from build123d import *

# Parameters (mm, degrees)
PAD007_DEPTH    = 14.7
PAD008_DEPTH    = 8.5
POCKET017_DEPTH = 7.22
SKETCH022_R     = 7.7
POCKET018_DEPTH = 26.5
SKETCH023_R     = 7.7
POCKET019_DEPTH = 26
SKETCH024_R     = 6
SKETCH024_R_2   = 5.5
POCKET020_DEPTH = 57.001
SKETCH025_R     = 7.7
POCKET021_DEPTH = 26
SKETCH020_W     = 25.7447
SKETCH020_H     = 35
POCKET022_DEPTH = 2.2
FILLET_R        = 1
FILLET001_R     = 1
FILLET002_R     = 2
SKETCH026_R     = 1.55
SKETCH026_R_2   = 1.6
POCKET023_DEPTH = 14.701
SKETCH027_R     = 1.55
POCKET024_DEPTH = 23.201
SKETCH028_R     = 1.55
POCKET025_DEPTH = 10
SKETCH029_W     = 10
SKETCH029_H     = 57
PAD009_DEPTH    = 9.5
POCKET026_DEPTH = 16.981
SKETCH031_W     = 10
SKETCH031_H     = 2.9
POCKET027_DEPTH = 1.5
POCKET028_DEPTH = 10
SKETCH033_R     = 1.7
POCKET029_DEPTH = 16
SKETCH_W        = 6
SKETCH_H        = 3
POCKET_DEPTH    = 23.201


with BuildPart() as part:
    # Sketch018 → Pad007 (new body)
    with BuildSketch(Plane.YZ):
        Polygon((0, 0), (0, 26), (-4.306836, 40.539634), (3.9, 57), (74.5, 57), (74.5, 0), align=None)
    extrude(amount=PAD007_DEPTH)

    # Sketch019 → Pad008 (new body)
    with BuildSketch(Plane.YZ.offset(14.7)):
        Polygon((19.7447, 57), (28.4947, 57), (28.4947, 12.3), (21.6234, 12.3), (21.6234, 26.5), (19.7447, 26.5), align=None)
    extrude(amount=PAD008_DEPTH)

    # Sketch021 → Pocket017 (cut)
    with BuildSketch(Plane.YZ.offset(14.7)):
        with BuildLine():
            ThreePointArc((44.6197, 57), (41.229345, 42.566333), (43.9947, 28))
            Line((43.9947, -6), (43.9947, 28))
            Line((43.9947, -6), (28.4947, -6))
            Line((28.4947, -6), (28.4947, 65))
            Line((28.4947, 65), (44.6197, 65))
            Line((44.6197, 65), (44.6197, 57))
        make_face()
    extrude(amount=-POCKET017_DEPTH, mode=Mode.SUBTRACT)

    # Sketch022 → Pocket018 (cut)
    with BuildSketch(Plane.YX):
        with Locations((14.25, 12.5)):
            Circle(SKETCH022_R)
    extrude(amount=-POCKET018_DEPTH, mode=Mode.SUBTRACT)

    # Sketch023 → Pocket019 (cut)
    with BuildSketch(Plane.YX):
        with Locations((59.25, 12.5)):
            Circle(SKETCH023_R)
    extrude(amount=-POCKET019_DEPTH, mode=Mode.SUBTRACT)

    # Sketch024 → Pocket020 (cut, through all)
    with BuildSketch(Plane(origin=(0, 0, 57), x_dir=(0, -1, 0), z_dir=(0, 0, 1))):
        with Locations((-59.25, 12.5)):
            Circle(SKETCH024_R)
        with Locations((-14.25, 12.5)):
            Circle(SKETCH024_R_2)
    extrude(amount=-POCKET020_DEPTH, mode=Mode.SUBTRACT)

    # Sketch025 → Pocket021 (cut)
    with BuildSketch(Plane(origin=(0, 0, 57), x_dir=(0, -1, 0), z_dir=(0, 0, 1))):
        with Locations((-59.25, 12.5)):
            Circle(SKETCH025_R)
    extrude(amount=-POCKET021_DEPTH, mode=Mode.SUBTRACT)

    # Sketch020 → Pocket022 (cut)
    with BuildSketch(Plane.YZ.offset(14.7)):
        with Locations((6.87235, 43.5)):
            Rectangle(SKETCH020_W, SKETCH020_H)
    extrude(amount=-POCKET022_DEPTH, mode=Mode.SUBTRACT)

    # Fillet
    fillet_edges = [part.edges().sort_by_distance(p)[0] for p in [
        (7.001325, 14.370727, 57),
        (7.001325, 14.370727, 26.5),
    ]]
    fillet(fillet_edges, radius=FILLET_R)

    # Fillet001
    fillet001_edges = [part.edges().sort_by_distance(p)[0] for p in [
        (6.25, 3.9, 57),
        (12.5, 5.825, 57),
        (12.5, -0.203418, 48.769817),
        (6.25, -4.306836, 40.539634),
        (12.5, -2.153418, 33.269817),
    ]]
    fillet(fillet001_edges, radius=FILLET001_R)

    # Fillet002
    fillet002_edges = [part.edges().sort_by_distance(p)[0] for p in [
        (7.35, 0, 0),
        (18.959389, 21.6234, 12.3),
        (11.09, 43.9947, 0),
        (11.09, 28.4947, 0),
        (7.35, 74.5, 0),
        (7.35, 74.5, 57),
        (11.09, 28.4947, 57),
        (18.95, 28.4947, 57),
    ]]
    fillet(fillet002_edges, radius=FILLET002_R)

    # Sketch026 → Pocket023 (cut, through all)
    with BuildSketch(Plane.YZ.offset(14.7)):
        with Locations((2, 40)):
            Circle(SKETCH026_R)
        with Locations((3.5, 19.8)):
            Circle(SKETCH026_R_2)
        with Locations((25, 6.2)):
            Circle(SKETCH026_R_2)
        with Locations((48.3, 44)):
            Circle(SKETCH026_R_2)
        with Locations((48.3, 13)):
            Circle(SKETCH026_R_2)
        with Locations((70.2, 44)):
            Circle(SKETCH026_R_2)
        with Locations((70.2, 13)):
            Circle(SKETCH026_R_2)
    extrude(amount=-POCKET023_DEPTH, mode=Mode.SUBTRACT)

    # Sketch027 → Pocket024 (cut, through all)
    with BuildSketch(Plane.YZ.offset(23.2)):
        with Locations((25, 40)):
            Circle(SKETCH027_R)
        with Locations((25, 17)):
            Circle(SKETCH027_R)
    extrude(amount=-POCKET024_DEPTH, mode=Mode.SUBTRACT)

    # Sketch028 → Pocket025 (cut)
    with BuildSketch(Plane(origin=(0, 19.7447, 0), x_dir=(0, 0, -1), z_dir=(0, -1, 0))):
        with Locations((-50.5, 19)):
            Circle(SKETCH028_R)
        with Locations((-31.5, 19)):
            Circle(SKETCH028_R)
    extrude(amount=-POCKET025_DEPTH, mode=Mode.SUBTRACT)

    # Sketch029 → Pad009 (new body)
    with BuildSketch(Plane.YZ.offset(7.48)):
        with Locations((35, 28.5)):
            Rectangle(SKETCH029_W, SKETCH029_H)
    extrude(amount=PAD009_DEPTH)

    # Sketch030 → Pocket026 (cut, through all)
    with BuildSketch(Plane.YZ.offset(16.98)):
        with BuildLine():
            Line((30, 49), (30, 57))
            Line((30, 57), (40, 57))
            Line((40, 57), (40, 49))
            Line((38.5, 49), (40, 49))
            ThreePointArc((35.5, 49), (37, 47.5), (38.5, 49))
            Line((34.5, 49), (35.5, 49))
            ThreePointArc((31.5, 49), (33, 47.5), (34.5, 49))
            Line((30, 49), (31.5, 49))
        make_face()
    extrude(amount=-POCKET026_DEPTH, mode=Mode.SUBTRACT)

    # Sketch031 → Pocket027 (cut)
    with BuildSketch(Plane(origin=(0, 0, 49), x_dir=(0, -1, 0), z_dir=(0, 0, 1))):
        with Locations((-35, 1.45)):
            Rectangle(SKETCH031_W, SKETCH031_H)
    extrude(amount=-POCKET027_DEPTH, mode=Mode.SUBTRACT)

    # Sketch032 → Pocket028 (cut)
    with BuildSketch(Plane.ZX.offset(40)):
        Polygon((0, 7.48), (0, 16.98), (47, 16.98), (35.678341, 7.48), align=None)
    extrude(amount=-POCKET028_DEPTH, mode=Mode.SUBTRACT)

    # Sketch033 → Pocket029 (cut)
    with BuildSketch(Plane(origin=(0, 0, 49), x_dir=(0, -1, 0), z_dir=(0, 0, 1))):
        with Locations((-35, 5.41526)):
            Circle(SKETCH033_R)
    extrude(amount=-POCKET029_DEPTH, mode=Mode.SUBTRACT)

    # Sketch → Pocket (cut, through all)
    with BuildSketch(Plane(origin=(0, 0, 0), x_dir=(0, 1, 0), z_dir=(-1, 0, 0))):
        with Locations((35, -40.5)):
            Rectangle(SKETCH_W, SKETCH_H)
    extrude(amount=-POCKET_DEPTH, mode=Mode.SUBTRACT)


solid = part.part
The listing builds one solid part. Answer for the finished solid, in the listing's coordinates (mm). A direction names the side the tool comes from. Round coordinates to 2 decimals unless told otherwise and drop trailing zeros. Loops run counter-clockwise (first coordinate to the right, second up) from the corner with the lowest first, then second, coordinate; pieces in that order, holes last. Notation, with made-up numbers: M 6,-16.75 L 56,-16.75 A23 cw 56,2.25 Z; hole C 79,64 d3. An arc over 180 degrees is marked long. Return JSON: item names as keys, results as strings.
Q1. The mould has two halves that part along Z. Classify faces 4 (the face through (10, 37, 47.5)), 5 (the face through (23.2, 24, 35)), 6 (the face through (7.45, 23.82, 7.28)): released by +Z, released by -Z, zero draft, split by the parting line, or undercut.
Results list:
{"face 4": "released by +Z", "face 5": "zero draft", "face 6": "undercut"}
Q2. Find the intervals of material crossed by line 1 along Z through (x, y) = (11.5, 70.2); line 2 along Z through (x, y) = (5.5, 33); line 3 along X through (y, z) = (3, 38.5), in increasing order. Write a range as from..to.
Results list:
{"line 1": "z = 0..11.4, 14.6..42.4, 45.6..57", "line 2": "z = 0..39, 42..47.5", "line 3": "x = 0..12.5"}
Q3. Each of these flat-tipped pins is pushed along its axis until it touches: pin 1 Ø3 at (x, z) = (20.5, 42) entering from +Y; pin 2 Ø3.5 at (y, z) = (3, 37.5) entering from +X; pin 3 Ø3 at (y, z) = (25, 6.2) entering from -X; pin 4 Ø4 at (y, z) = (29.5, 38) entering from +X. Where does it stop, or does it pass through?
Results list:
{"pin 1": "stops at y = 28.49", "pin 2": "stops at x = 12.5", "pin 3": "passes through", "pin 4": "stops at x = 23.2"}
Q4. Find section B-B, the plane y = 25. Determine the outline of the cut face in (x, z), plus the area to 3 significant figures.
Results list:
{"outline": "M 0,0 L 14.7,0 L 14.7,4.6 L 0,4.6 Z; M 0,7.8 L 14.7,7.8 L 14.7,12.3 L 23.2,12.3 L 23.2,15.45 L 0,15.45 Z; M 0,18.55 L 23.2,18.55 L 23.2,38.45 L 0,38.45 Z; M 0,41.55 L 23.2,41.55 L 23.2,57 L 0,57 Z; hole C 19,31.5 d3.1; hole C 19,50.5 d3.1", "area": "1,010 mm2"}
Q5. Find section D-D, the plane x = 9. State how many separate pieces and enclosed holes the cut face has, plus the area to 3 significant figures.
Results list:
{"separate pieces": "5", "enclosed holes": "10", "area": "2,080 mm2"}
Q6. Find section A-A, the plane y = 48.3. Determine the outline of the cut face in (x, z).
Results list:
{"outline": "M 0,0 L 14.7,0 L 14.7,11.4 L 0,11.4 Z; M 0,14.6 L 14.7,14.6 L 14.7,42.4 L 0,42.4 Z; M 0,45.6 L 14.7,45.6 L 14.7,57 L 0,57 Z"}
Q7. Find section C-C, the plane z = 6.2. Determine the outline of the cut face in (x, y), plus the area to 3 significant figures.
Results list:
{"outline": "M 0,0 L 14.7,0 L 14.7,6.87 A7.7 cw long 14.7,21.63 L 14.7,23.4 L 0,23.4 Z; M 0,26.6 L 14.7,26.6 L 14.7,28.49 L 7.48,28.49 L 7.48,43.99 L 14.7,43.99 L 14.7,51.87 A7.7 cw long 14.7,66.63 L 14.7,74.5 L 0,74.5 Z", "area": "683 mm2"}
Q8. Which of the six approach directions +Z, -Z, +X, -X, +Y, -Y give full straight-line access (tool end or side, diameter ignored) to faces 1 (the face through (10, 31, 49)), 2 (the face through (19.01, 22.194, 12.901)), 3 (the face through (2.9, 31, 48))?
Results list:
{"face 1": "+Z, +X, -X", "face 2": "-Z, +X, -Y", "face 3": "+Z, -X"}
